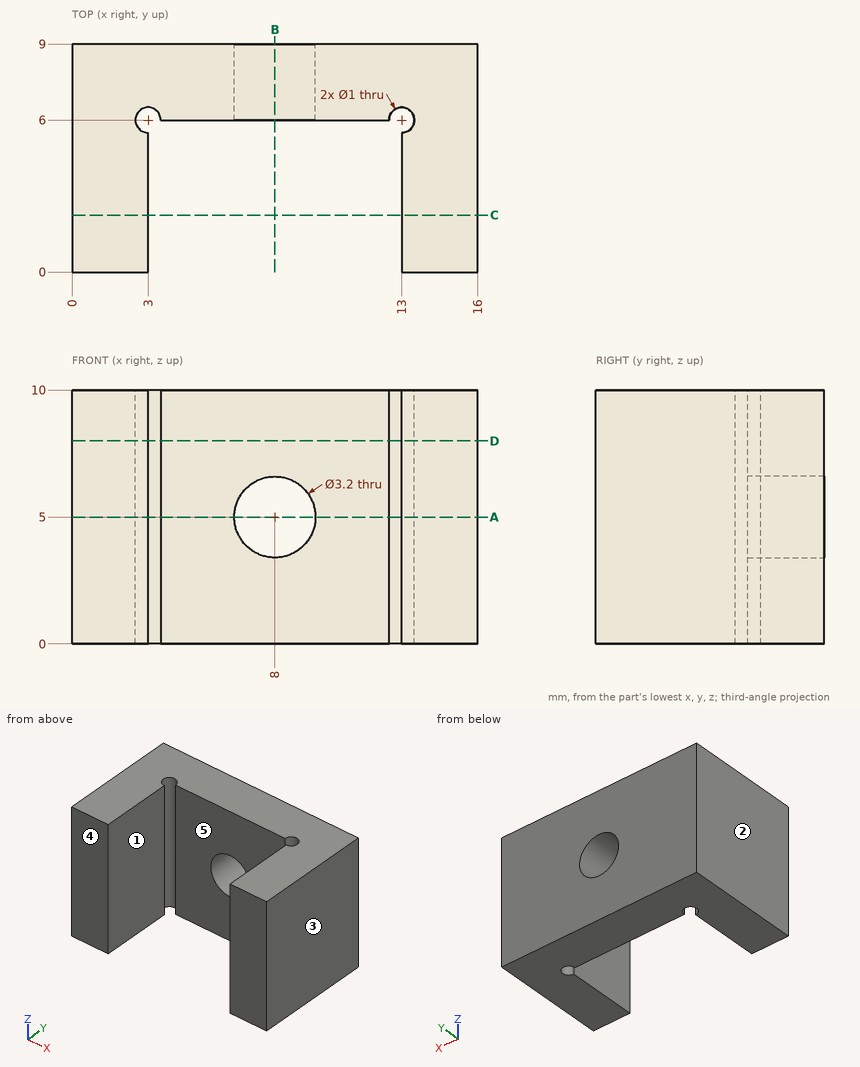
Print and shaded views of the part. All mm, measured from the part's lowest x, y and z. A direction names the side the tool comes from. Coordinates: 2 decimals unless noted, no trailing zeros. Loops run counter-clockwise (first coordinate to the right, second up) from the corner with the lowest first, then second, coordinate; pieces in that order, holes last. Notation, with made-up numbers: M 83.25,22.25 L 129.25,22.25 A31 cw 129.25,58.25 Z; hole C 70.5,75 d8. An arc over 180 degrees is marked long. Use a Markdown table: item, result. Add a question column.
Q1. Probe L1, parallel to X at y = 3.5, z = 9.5; L2, parallel to X at y = 7.95, z = 5; L3, parallel to Y at x = 11.75, z = 1.5. List the from-to ranges inside material, lowest first.
Q2. Which spindle directions (+Z, -Z, +X, -X, +Y, -Y) get a long thin tool onto all of the face, cutting with end or side? Do the marked faces 1 and 2. Say none if no direction does.
Q3. Pin check, flat tips, straight feed: P1, Ø1, axis at x = 10.5, z = 5.5, coming from the -Y side; P2, Ø3, axis at x = 8, y = 4, coming from the -Z side. Stop position of each tip, or through.
Q4. Cut at D-D (z = 8). Write the cut outline in (x, y), and give its area (3 significant figures).
Q5. Cut at B-B (x = 8). Write the cut outline in (y, z), and give its area (3 significant figures).
Q6. Cut at C-C (y = 2.25). Write the cut outline in (x, z), and give its area (3 significant figures).
Q7. Mould opens along X. For the marked faces 3, 4 and 5 say: +X half, -X half, draft (parallel to the pull), parting line (faces both ways), or undercut.
Q8. Cut at A-A (z = 5). Write the cut outline in (x, y).
Worked out:
| question | item | result |
|---|---|---|
| 1 | L1 | x = 0 to 3, 13 to 16 |
| 1 | L2 | x = 0 to 6.4, 9.6 to 16 |
| 1 | L3 | y = 6 to 9 |
| 2 | face 1 | +Z, -Z, -Y |
| 2 | face 2 | +Z, -Z, -X, +Y, -Y |
| 3 | P1 | stops at y = 6 |
| 3 | P2 | passes through |
| 4 | outline | M 0,0 L 3,0 L 3,5.5 A0.5 cw long 3.5,6 L 12.5,6 A0.5 cw long 13,5.5 L 13,0 L 16,0 L 16,9 L 0,9 Z |
| 4 | area | 82.8 mm2 |
| 5 | outline | M 6,0 L 9,0 L 9,3.4 L 6,3.4 Z; M 6,6.6 L 9,6.6 L 9,10 L 6,10 Z |
| 5 | area | 20.4 mm2 |
| 6 | outline | M 0,0 L 3,0 L 3,10 L 0,10 Z; M 13,0 L 16,0 L 16,10 L 13,10 Z |
| 6 | area | 60.0 mm2 |
| 7 | face 3 | +X half |
| 7 | face 4 | draft |
| 7 | face 5 | undercut |
| 8 | outline | M 0,0 L 3,0 L 3,5.5 A0.5 cw long 3.5,6 L 6.4,6 L 6.4,9 L 0,9 Z; M 9.6,6 L 12.5,6 A0.5 cw long 13,5.5 L 13,0 L 16,0 L 16,9 L 9.6,9 Z |
